from build123d import *

# Parameters (mm, degrees)
F1_DEPTH = 12.7
F2_R     = 25.4


with BuildPart() as f1:
    # F0 (on Front) → F1 (new body)
    with BuildSketch(Plane.XZ):
        Polygon((76.2, 220.150558), (0, 220.150558), (-76.2, 220.150558), (-304.8, -1151.449442), (0, -1151.449442), (304.8, -1151.449442), align=None)
        Polygon((230.390112, -1091.245532), (0, -1091.245532), (-230.390112, -1091.245532), (-168.45743, -719.649442), (0, -719.649442), (168.45743, -719.649442), align=None, mode=Mode.SUBTRACT)
        Polygon((157.874097, -656.149442), (0, -656.149442), (-157.874097, -656.149442), (-96.490763, -287.849442), (0, -287.849442), (96.490763, -287.849442), align=None, mode=Mode.SUBTRACT)
        Polygon((85.90743, -224.349442), (0, -224.349442), (-85.90743, -224.349442), (-22.40743, 156.650558), (0, 156.650558), (22.40743, 156.650558), align=None, mode=Mode.SUBTRACT)
    extrude(amount=F1_DEPTH)

    # F2
    f2_edges = [f1.edges().sort_by_distance(p)[0] for p in [
        (-85.90743, -6.35, -224.349442),
        (85.90743, -6.35, -224.349442),
        (22.40743, -6.35, 156.650558),
        (-22.40743, -6.35, 156.650558),
        (-96.490763, -6.35, -287.849442),
        (96.490763, -6.35, -287.849442),
        (157.874097, -6.35, -656.149442),
        (-157.874097, -6.35, -656.149442),
        (-230.390112, -6.35, -1091.245532),
        (168.45743, -6.35, -719.649442),
        (230.390112, -6.35, -1091.245532),
        (-168.45743, -6.35, -719.649442),
    ]]
    fillet(f2_edges, radius=F2_R)


solid = f1.part
The model under review builds one solid part; all positions refer to its coordinate system, in mm. A direction names the side the tool comes from. Coordinates: 2 decimals unless noted, no trailing zeros. Loops run counter-clockwise (first coordinate to the right, second up) from the corner with the lowest first, then second, coordinate; pieces in that order, holes last. Notation, with made-up numbers: (67.25, -25.5) -> (82.25, -25.5) arc R18 ccw to (82.25, -7.5) -> close; hole circle Ø9 at (-26.5, 10). An arc over 180 degrees is marked (long way). Use a Markdown table: item, result. Add a question column.
1. Add section C-C on z = -119.5. Write out the cut boundary in (x, y), plus the area to 3 significant figures.
2. Clearance check with flat-ended pins moving along their axes: pin 1 Ø1 at (y, z) = (-7, -35.5) entering from -X; pin 2 Ø5 at (y, z) = (-6.5, -448) entering from -X; pin 3 Ø2 at (y, z) = (-6, -839.5) entering from -X. State where each tip first meets the part, or that it passes through.
3. Draft analysis for pull direction X (two halves, no side actions). For faces 3 (the face through (-75.104, -6.439, -215.602)), 4 (the face through (-188.9, -6.26, -456.05)), 5 (the face through (-1, 0, -666)), state which applies: pulls with the +X half, pulls with the -X half, needs draft (parallel to the pull), parting line crosses it, or undercut.
4. Add section A-A on y = -5.25. Write out the cut boundary in (x, z), plus the area to 3 significant figures.
5. Add section B-B on x = 186. Write out the cut boundary in (y, z), plus the area to 3 significant figures.
6. Machinability: for faces 1 (the face through (192.1, -6.26, -475.25)), 2 (the face through (53.076, -6.261, -27.362)), which of the approach directions +Z, -Z, +X, -X, +Y, -Y give a long, thin tool a straight path to every point of the face, cutting with its end or side? Answer none if there is none.
7. To check wall thickness, follow line 1 (Z direction, x = -13, y = -11.75); line 2 (Z direction, x = -21.5, y = -6.5); line 3 (X direction, y = -4.25, z = -1057.5). State the ranges of each line that lie inside material, in increasing order.
Returned:
| question | item | result |
|---|---|---|
| 1 | outline | (-132.81, -12.7) -> (-68.43, -12.7) -> (-68.43, 0) -> (-132.81, 0) -> close; (68.43, -12.7) -> (132.81, -12.7) -> (132.81, 0) -> (68.43, 0) -> close |
| 1 | area | 1,640 mm² |
| 2 | pin 1 | stops at x = -118.89 |
| 2 | pin 2 | stops at x = -187.98 |
| 2 | pin 3 | stops at x = -252.98 |
| 3 | face 3 | undercut |
| 3 | face 4 | pulls with the -X half |
| 3 | face 5 | needs draft |
| 4 | outline | (-304.8, -1151.45) -> (304.8, -1151.45) -> (76.2, 220.15) -> (-76.2, 220.15) -> close; hole (-225.46, -1061.67) arc R25.4 ccw to (-200.41, -1091.25) -> (200.41, -1091.25) arc R25.4 ccw to (225.46, -1061.67) -> (171.99, -740.87) arc R25.4 ccw to (146.94, -719.65) -> (-146.94, -719.65) arc R25.4 ccw to (-171.99, -740.87) -> close; hole (-152.94, -626.57) arc R25.4 ccw to (-127.89, -656.15) -> (127.89, -656.15) arc R25.4 ccw to (152.94, -626.57) -> (100.03, -309.07) arc R25.4 ccw to (74.97, -287.85) -> (-74.97, -287.85) arc R25.4 ccw to (-100.03, -309.07) -> close; hole (-80.98, -194.77) arc R25.4 ccw to (-55.92, -224.35) -> (55.92, -224.35) arc R25.4 ccw to (80.98, -194.77) -> (25.94, 135.43) arc R25.4 ccw to (0.89, 156.65) -> (-0.89, 156.65) arc R25.4 ccw to (-25.94, 135.43) -> close |
| 4 | area | 241,000 mm² |
| 5 | outline | (-12.7, -1151.45) -> (0, -1151.45) -> (0, -1091.25) -> (-12.7, -1091.25) -> close; (-12.7, -824.9) -> (0, -824.9) -> (0, -438.65) -> (-12.7, -438.65) -> close |
| 5 | area | 5,670 mm² |
| 6 | face 1 | +Z, +X, +Y, -Y |
| 6 | face 2 | +Y, -Y |
| 7 | line 1 | z = -1151.45 to -1091.25, -719.65 to -656.15, -287.85 to -224.35, 153.58 to 220.15 |
| 7 | line 2 | z = -1151.45 to -1091.25, -719.65 to -656.15, -287.85 to -224.35, 146.1 to 220.15 |
| 7 | line 3 | x = -289.14 to -224.77, 224.77 to 289.14 |
